```python
from build123d import *

# Parameters (mm, degrees)
ESQUISSE1_W                                   = 30
ESQUISSE1_H                                   = 30
ESQUISSE1_R                                   = 12
BOSS_EXTRU_1_DEPTH                            = 6
ESQUISSE2_R                                   = 13
ENL_V_MAT_EXTRU_1_DEPTH                       = 5
TROU_POUR_TARAUDAGE_POUR_TROU_TARAUD_M3_D     = 2.5
TROU_POUR_TARAUDAGE_POUR_TROU_TARAUD_M3_DEPTH = 6
TROU_POUR_TARAUDAGE_POUR_TROU_TARAUD_M3_TIP   = 0.751075774
TROU_POUR_TARAUDAGE_POUR_TROU_TARAUD_2_D      = 2.5
TROU_POUR_TARAUDAGE_POUR_TROU_TARAUD_2_DEPTH  = 6
TROU_POUR_TARAUDAGE_POUR_TROU_TARAUD_2_TIP    = 0.751075774
CONG_1_R                                      = 0.3


with BuildPart() as part:
    # Esquisse1 → Boss.-Extru.1 (new body)
    with BuildSketch(Plane.XY):
        with Locations((15, 15)):
            Rectangle(ESQUISSE1_W, ESQUISSE1_H)
        with Locations((15, 15)):
            Circle(ESQUISSE1_R, mode=Mode.SUBTRACT)
    extrude(amount=BOSS_EXTRU_1_DEPTH)

    # Esquisse2 → Enlèv. mat.-Extru.1 (cut)
    with BuildSketch(Plane.XY.offset(6)):
        with Locations((15, 15)):
            Circle(ESQUISSE2_R)
    extrude(amount=-ENL_V_MAT_EXTRU_1_DEPTH, mode=Mode.SUBTRACT)

    # Trou pour taraudage pour trou taraud_ M3
    with Locations(Plane(origin=(0, 30, 0), x_dir=(1, 0, 0), z_dir=(0, 1, 0))):
        with Locations((3, -3), (27, -3)):
            Hole(TROU_POUR_TARAUDAGE_POUR_TROU_TARAUD_M3_D / 2, depth=TROU_POUR_TARAUDAGE_POUR_TROU_TARAUD_M3_DEPTH)
            with Locations((0, 0, -(TROU_POUR_TARAUDAGE_POUR_TROU_TARAUD_M3_DEPTH + TROU_POUR_TARAUDAGE_POUR_TROU_TARAUD_M3_TIP / 2))):  # 118° drill point
                Cone(0, TROU_POUR_TARAUDAGE_POUR_TROU_TARAUD_M3_D / 2, TROU_POUR_TARAUDAGE_POUR_TROU_TARAUD_M3_TIP, mode=Mode.SUBTRACT)

    # Trou pour taraudage pour trou taraud 2
    with Locations(Plane(origin=(0, 0, 0), x_dir=(-1, 0, 0), z_dir=(0, -1, 0))):
        with Locations((-3, -3), (-27, -3)):
            Hole(TROU_POUR_TARAUDAGE_POUR_TROU_TARAUD_2_D / 2, depth=TROU_POUR_TARAUDAGE_POUR_TROU_TARAUD_2_DEPTH)
            with Locations((0, 0, -(TROU_POUR_TARAUDAGE_POUR_TROU_TARAUD_2_DEPTH + TROU_POUR_TARAUDAGE_POUR_TROU_TARAUD_2_TIP / 2))):  # 118° drill point
                Cone(0, TROU_POUR_TARAUDAGE_POUR_TROU_TARAUD_2_D / 2, TROU_POUR_TARAUDAGE_POUR_TROU_TARAUD_2_TIP, mode=Mode.SUBTRACT)

    # Congé1
    cong_1_edges = [part.edges().sort_by_distance(p)[0] for p in [
        (0, 30, 3),
        (30, 30, 3),
        (30, 0, 3),
        (0, 0, 3),
    ]]
    fillet(cong_1_edges, radius=CONG_1_R)


solid = part.part
```
Geometry: final body of the model. Coordinates: model frame, mm. A direction names the side the tool comes from. Coordinates: 2 decimals unless noted, no trailing zeros. Loops run counter-clockwise (first coordinate to the right, second up) from the corner with the lowest first, then second, coordinate; pieces in that order, holes last. Notation, with made-up numbers: (-11, 45) -> (13, 45) arc R24 ccw to (13, 80) -> close; hole circle Ø1 at (-22, 20). An arc over 180 degrees is marked (long way). Use a Markdown table: item, result. Add a question column.
(1) Section query A-A, the plane y = 15. Return loops of the section in (x, z).
(2) Access query for faces 5 (the cylindrical face through (1.81, 26.96, 2.62)), 6 (the cylindrical face through (27.4, 18.9, 3.5)), 7 (the cylindrical face through (28.155, 3.042, 3.479)). Directions: +Z, -Z, +X, -X, +Y, -Y. A direction counts if a zero-diameter tool reaches every point of the face in a straight line with its end or side. Return the directions, or none.
(3) Section query C-C, the plane z = 0.4. Return loops of the section in (x, y).
(4) Line query: line 1 along Z through (x, y) = (3, 4.55); line 2 along X through (y, z) = (15, 0.3); line 3 along Z through (x, y) = (26.25, 9.75). Output: solid intervals per line, ascending.
(5) Mould query, pull axis Z, two halves, no side actions, for faces 1 (the cylindrical face through (25.845, 26.958, 3.479)), 2 (the flat face through (24, 6, 1)), 3 (the flat face through (8, 25, 0)), 4 (the flat face through (0, 15, 3)). Classes: pulls with the +Z half, pulls with the -Z half, needs draft (parallel to the pull), parting line crosses it, or undercut.
(6) Section query D-D, the plane y = 27.5. Return loops of the section in (x, z), plus the area to 3 significant figures.
(7) Pin query (flat end, axial travel): pin 1 Ø1.5 at (x, z) = (3, 3) entering from -Y; pin 2 Ø2 at (x, z) = (27, 3) entering from +Y. Return the tip coordinate at first contact, or that it passes through.
Answer:
| question | item | result |
|---|---|---|
| 1 | outline | (0, 0) -> (3, 0) -> (3, 1) -> (2, 1) -> (2, 6) -> (0, 6) -> close; (27, 0) -> (30, 0) -> (30, 6) -> (28, 6) -> (28, 1) -> (27, 1) -> close |
| 2 | face 5 | +Y |
| 2 | face 6 | +Z |
| 2 | face 7 | -Y |
| 3 | outline | (0, 0.3) arc R0.3 ccw to (0.3, 0) -> (29.7, 0) arc R0.3 ccw to (30, 0.3) -> (30, 29.7) arc R0.3 ccw to (29.7, 30) -> (0.3, 30) arc R0.3 ccw to (0, 29.7) -> close; hole circle Ø24 at (15, 15) |
| 4 | line 1 | z = 0 to 1.75, 4.25 to 6 |
| 4 | line 2 | x = 0 to 3, 27 to 30 |
| 4 | line 3 | z = 0 to 1 |
| 5 | face 1 | undercut |
| 5 | face 2 | pulls with the +Z half |
| 5 | face 3 | pulls with the -Z half |
| 5 | face 4 | needs draft |
| 6 | outline | (0, 0) -> (30, 0) -> (30, 6) -> (18.57, 6) -> (18.57, 1) -> (11.43, 1) -> (11.43, 6) -> (0, 6) -> close; hole circle Ø2.5 at (3, 3); hole circle Ø2.5 at (27, 3) |
| 6 | area | 134 mm^2 |
| 7 | pin 1 | stops at y = 6.3 |
| 7 | pin 2 | stops at y = 23.85 |
